Read the model definition and answer for the solid it produces. Units are mm, in the model's axes. A direction names the side the tool comes from. Round coordinates to 2 decimals unless told otherwise and drop trailing zeros. Loops run counter-clockwise (first coordinate to the right, second up) from the corner with the lowest first, then second, coordinate; pieces in that order, holes last. Notation, with made-up numbers: M -12,89.25 L 1,89.25 A22 ccw 1,95.25 Z; hole C -26.75,-16.5 d4. An arc over 180 degrees is marked long. Write each question's results on one line, items separated by ' | '.
Autodesk Inventor part; units mm, degrees
ref_plane "YZ Plane" through (0, 0, 0) normal (1, 0, 0) x (0, 1, 0)
ref_plane "XZ Plane" through (0, 0, 0) normal (0, 1, 0) x (-1, 0, 0)
ref_plane "XY Plane" through (0, 0, 0) normal (0, 0, 1) x (1, 0, 0)
sketch "草图1" plane through (0, 0, 0) normal (0, 0, 1) x (1, 0, 0)
  line L0 (32.05, -44.65) -> (-32.05, -44.65)
  line L1 (-32.05, -44.65) -> (-32.05, 44.65)
  line L2 (-32.05, 44.65) -> (32.05, 44.65)
  line L3 (32.05, 44.65) -> (32.05, -44.65)
  line L4 (32.05, -44.65) -> (-32.05, 44.65) construction
  line L5 (-32.05, -44.65) -> (32.05, 44.65) construction
  line L6 (24.111, -19.563) -> (-24.389, -19.563) construction
  line L7 (-24.389, -19.563) -> (-24.389, 4.437) construction
  line L8 (-24.389, 4.437) -> (24.111, 4.437) construction
  line L9 (24.111, 4.437) -> (24.111, -19.563) construction
  line L10 (24.111, -19.563) -> (-24.389, 4.437) construction
  line L11 (-24.389, -19.563) -> (24.111, 4.437) construction
  circle A0 centre (-24.389, 4.437) radius 1.7
  circle A1 centre (-24.389, -19.563) radius 1.7
  circle A2 centre (24.111, 4.437) radius 1.7
  circle A3 centre (24.111, -19.563) radius 1.7
  line L12 (29.55, -43.15) -> (-4.45, -43.15)
  line L13 (-4.45, -43.15) -> (-4.45, -38.15)
  line L14 (-4.45, -38.15) -> (29.55, -38.15)
  line L15 (29.55, -38.15) -> (29.55, -43.15)
  line L16 (-19.55, -38.15) -> (-7.55, -38.15)
  line L17 (-7.55, -38.15) -> (-7.55, -33.65)
  line L18 (-7.55, -33.65) -> (-19.55, -33.65)
  line L19 (-19.55, -33.65) -> (-19.55, -38.15)
  line L20 (-20.05, -32.65) -> (-29.05, -32.65)
  line L21 (-29.05, -32.65) -> (-29.05, -28.15)
  line L22 (-29.05, -28.15) -> (-20.05, -28.15)
  line L23 (-20.05, -28.15) -> (-20.05, -32.65)
  line L24 (-12.05, 20.15) -> (-0.05, 20.15)
  line L25 (-0.05, 20.15) -> (-0.05, 24.65)
  line L26 (-0.05, 24.65) -> (-12.05, 24.65)
  line L27 (-12.05, 24.65) -> (-12.05, 20.15)
  point P0 (0, 0)
  point P1 (-0.139, -7.563)
  point P2 (-20.05, -30.4)
  dimension "d0" = 64.1
  dimension "d1" = 89.3
  dimension "d2" = 48.5
  dimension "d3" = 24
  dimension "d4" = 52.213
  dimension "d5" = 37.087
  dimension "d6" = 32.189
  dimension "d7" = 31.911
  dimension "d8" = 3.4
  dimension "d16" = 6.5
  dimension "d20" = 24.5
  dimension "d21" = 36.5
  dimension "d22" = 12.5
  dimension "d23" = 11
  dimension "d24" = 6.5
  dimension "d25" = 2.5
  dimension "d26" = 1.5
  dimension "d27" = 12
  dimension "d28" = 12
  dimension "d29" = 3
  dimension "d30" = 16.5
  dimension "d31" = 32
  dimension "d32" = 20
  dimension "d33" = 24.5
  dimension "d34" = 20
extrude "拉伸1" add sketch "草图1" along normal blind 2
sketch "草图5" plane through (0, 0, 0) normal (0, 0, -1) x (-1, 0, 0)
  circle A0 centre (24.389, -19.563) radius 1.7
  circle A1 centre (24.389, -19.563) radius 3
  circle A2 centre (24.389, 4.437) radius 1.7
  circle A3 centre (24.389, 4.437) radius 3
  circle A4 centre (-24.111, -19.563) radius 1.7
  circle A5 centre (-24.111, -19.563) radius 3
  circle A6 centre (-24.111, 4.437) radius 1.7
  circle A7 centre (-24.111, 4.437) radius 3
  line L0 (-32.05, 44.65) -> (32.05, 44.65)
  line L1 (32.05, -44.65) -> (-32.05, -44.65)
  line L2 (-32.05, -44.65) -> (-32.05, 44.65)
  line L3 (-32.05, 44.65) -> (32.05, 44.65)
  line L4 (32.05, 44.65) -> (32.05, -44.65)
  line L5 (20.05, -32.65) -> (29.05, -32.65)
  line L6 (29.05, -28.15) -> (20.05, -28.15)
  line L7 (29.05, -32.65) -> (20.05, -32.65)
  line L8 (20.05, -32.65) -> (20.05, -28.15)
  line L9 (20.05, -28.15) -> (29.05, -28.15)
  line L10 (29.05, -28.15) -> (29.05, -32.65)
  line L11 (7.55, -38.15) -> (19.55, -38.15)
  line L12 (19.55, -38.15) -> (7.55, -38.15)
  line L13 (7.55, -38.15) -> (7.55, -33.65)
  line L14 (7.55, -33.65) -> (19.55, -33.65)
  line L15 (19.55, -33.65) -> (19.55, -38.15)
  line L16 (4.45, -43.15) -> (4.45, -38.15)
  line L17 (-29.55, -38.15) -> (-29.55, -43.15)
  line L18 (4.45, -43.15) -> (-29.55, -43.15)
  line L19 (-29.55, -43.15) -> (-29.55, -38.15)
  line L20 (-29.55, -38.15) -> (4.45, -38.15)
  line L21 (4.45, -38.15) -> (4.45, -43.15)
  line L22 (12.05, 24.65) -> (0.05, 24.65)
  line L23 (12.05, 20.15) -> (0.05, 20.15)
  line L24 (0.05, 20.15) -> (0.05, 24.65)
  line L25 (0.05, 24.65) -> (12.05, 24.65)
  line L26 (12.05, 24.65) -> (12.05, 20.15)
  point P0 (0, 0)
  dimension "d48" = 6
  dimension "d49" = 6
  dimension "d50" = 6
  dimension "d51" = 6
extrude "拉伸5" add sketch "草图5" along normal blind 1 contours L0 L4 L1 L2
sketch "草图6" plane through (0, 0, -1) normal (0, 0, -1) x (-1, 0, 0)
  line L0 (-32.05, 44.65) -> (32.05, 44.65)
  line L1 (32.05, -44.65) -> (-32.05, -44.65)
  line L2 (-32.05, -44.65) -> (-32.05, 44.65)
  line L3 (-32.05, 44.65) -> (32.05, 44.65)
  line L4 (32.05, 44.65) -> (32.05, -44.65)
  circle A0 centre (24.389, -19.563) radius 3
  circle A1 centre (24.389, -19.563) radius 3
  circle A2 centre (24.389, 4.437) radius 3
  circle A3 centre (24.389, 4.437) radius 3
  circle A4 centre (-24.111, -19.563) radius 1.7
  circle A5 centre (-24.111, -19.563) radius 3
  circle A6 centre (-24.111, 4.437) radius 1.7
  circle A7 centre (-24.111, 4.437) radius 3
  point P0 (0, 0)
extrude "拉伸6" add sketch "草图6" along normal blind 1 contours L0 L4 L1 L2
sketch "草图7" plane through (0, 0, 2) normal (0, 0, 1) x (1, 0, 0)
  line L0 (32.05, 44.65) -> (-32.05, 44.65) construction
  line L1 (32.05, 44.65) -> (-32.05, 44.65) construction
  line L2 (-32.05, 44.65) -> (-32.05, -44.65) construction
  line L3 (-32.05, -44.65) -> (32.05, -44.65) construction
  line L4 (32.05, -44.65) -> (32.05, 44.65) construction
  line L5 (-27.55, 40.65) -> (-21.05, 40.65)
  line L6 (-21.05, 40.65) -> (-21.05, 23.15)
  line L7 (-21.05, 23.15) -> (-27.55, 23.15)
  line L8 (-27.55, 23.15) -> (-27.55, 40.65)
  point P0 (0, 0)
  point P1 (-21.05, 31.9)
  dimension "d56" = 4.5
  dimension "d58" = 4
  dimension "d59" = 21.5
  dimension "d68" = 6.5
extrude "拉伸7" cut sketch "草图7" against normal blind 3
sketch "草图8" plane through (0, 0, -2) normal (0, 0, -1) x (-1, 0, 0)
  line L0 (32.05, 44.65) -> (32.05, -44.65)
  line L1 (-32.05, -44.65) -> (-32.05, 44.65)
  line L2 (32.05, 44.65) -> (-32.05, 44.65)
  line L3 (-32.05, 44.65) -> (-32.05, -44.65)
  line L4 (-32.05, -44.65) -> (32.05, -44.65)
  line L5 (32.05, -44.65) -> (32.05, 44.65)
  line L6 (-32.55, 45.15) -> (32.55, 45.15)
  line L7 (32.55, 45.15) -> (32.55, -45.15)
  line L8 (32.55, -45.15) -> (-32.55, -45.15)
  line L9 (-32.55, -45.15) -> (-32.55, 45.15)
  point P0 (0, 0)
  dimension "d62" = 0.5
extrude "拉伸8" add sketch "草图8" against normal up to surface (4 mm away)
sketch "草图9" plane through (0, 0, -2) normal (0, 0, -1) x (-1, 0, 0)
  line L0 (-32.55, 45.15) -> (-32.55, -45.15)
  line L1 (32.55, -45.15) -> (32.55, 45.15)
  line L2 (-32.55, 45.15) -> (32.55, 45.15)
  line L3 (32.55, 45.15) -> (32.55, -45.15)
  line L4 (32.55, -45.15) -> (-32.55, -45.15)
  line L5 (-32.55, -45.15) -> (-32.55, 45.15)
  line L6 (33.55, 46.15) -> (-33.55, 46.15)
  line L7 (-33.55, 46.15) -> (-33.55, -46.15)
  line L8 (-33.55, -46.15) -> (33.55, -46.15)
  line L9 (33.55, -46.15) -> (33.55, 46.15)
  point P0 (0, 0)
  dimension "d65" = 1
extrude "拉伸9" add sketch "草图9" against normal blind 5.5
properties part number "TES_ESP32-Case"
Item 1: Flat-ended cylindrical pins translate along their axes: pin 1 (3.5 mm diameter, centred on x = -6.5, y = 23, fed in from +Z); pin 2 (1.5 mm diameter, centred on x = -26.5, y = -19.5, fed in from -Z); pin 3 (2 mm diameter, centred on x = -25.5, y = 33.5, fed in from +Z). Find the tip coordinate at first contact, or state that the pin passes through.
Outcome:
pin 1: stops at z = 2 | pin 2: stops at z = 0 | pin 3: stops at z = -1
Item 2: The part is cut by section C-C (z = 1.15). State how many separate pieces and enclosed holes the cut face has, plus the area to 3 significant figures.
Outcome:
separate pieces: 1 | enclosed holes: 9 | area: 5,720 mm2
Item 3: The part is cut by section D-D (y = -14). Determine the outline of the cut face in (x, z).
Outcome:
outline: M -33.55,-2 L 33.55,-2 L 33.55,3.5 L 32.55,3.5 L 32.55,2 L -32.55,2 L -32.55,3.5 L -33.55,3.5 Z
Item 4: Straight lines are drawn through the part: line 1 (Y direction, x = -0.5, z = -0.4); line 2 (Y direction, x = -3, z = 2.9); line 3 (X direction, y = 33, z = 0.35). For each, find the intervals that lie inside material, in ascending order.
Outcome:
line 1: y = -46.15 to -43.15, -38.15 to 20.15, 24.65 to 46.15 | line 2: y = -46.15 to -45.15, 45.15 to 46.15 | line 3: x = -33.55 to -27.55, -21.05 to 33.55
Item 5: For faces 4 (the face through (-20.05, -30, 0)), 5 (the face through (25.4, 3.1, 0)), 6 (the face through (-26.087, 4.362, 0.986)), determine the directions among +Z, -Z, +X, -X, +Y, -Y from which every point of the face is accessible in a straight line to the end or side of a thin tool.
Outcome:
face 4: +Z | face 5: -Z | face 6: +Z, -Z
Item 6: The part is cut by section B-B (x = -16). Determine the outline of the cut face in (y, z), plus the area to 3 significant figures.
Outcome:
outline: M -46.15,-2 L 46.15,-2 L 46.15,3.5 L 45.15,3.5 L 45.15,2 L -33.65,2 L -33.65,-1 L -38.15,-1 L -38.15,2 L -45.15,2 L -45.15,3.5 L -46.15,3.5 Z | area: 359 mm2
Item 7: The part is cut by section A-A (y = 31.5). Determine the outline of the cut face in (x, z).
Outcome:
outline: M -33.55,-2 L 33.55,-2 L 33.55,3.5 L 32.55,3.5 L 32.55,2 L -21.05,2 L -21.05,-1 L -27.55,-1 L -27.55,2 L -32.55,2 L -32.55,3.5 L -33.55,3.5 Z
Item 8: The mould has two halves that part along X. Classify faces 1 (the face through (21.34, -18.41, -0.99)), 2 (the face through (-25, -28.15, 0)), 3 (the face through (0, 46.15, 1)): pulls with the +X half, pulls with the -X half, needs draft (parallel to the pull), parting line crosses it, or undercut.
Outcome:
face 1: undercut | face 2: undercut | face 3: needs draft
